```python
from build123d import *

# Parameters (mm, degrees)
SKETCH2_W           = 12
SKETCH2_H           = 40
BOSS_EXTRUDE1_DEPTH = 5
SKETCH3_W           = 12.004104261
SKETCH3_H           = 2.6
CUT_EXTRUDE1_DEPTH  = 15
SKETCH4_W           = 12
SKETCH4_H           = 4
BOSS_EXTRUDE2_DEPTH = 15
SKETCH5_R           = 3.75
CUT_EXTRUDE2_DEPTH  = 15


with BuildPart() as part:
    # Sketch2 → Boss-Extrude1 (new body)
    with BuildSketch(Plane(origin=(0, 0, 0), x_dir=(1, 0, 0), z_dir=(0, 1, 0))):
        with Locations((-9.764705882, 23.058823529)):
            Rectangle(SKETCH2_W, SKETCH2_H)
    extrude(amount=BOSS_EXTRUDE1_DEPTH)

    # Sketch3 → Cut-Extrude1 (cut)
    with BuildSketch(Plane.XY.offset(-3.058823529)):
        with Locations((-9.766758013, 2.489565118)):
            Rectangle(SKETCH3_W, SKETCH3_H)
    extrude(amount=-CUT_EXTRUDE1_DEPTH, mode=Mode.SUBTRACT)

    # Sketch4 → Boss-Extrude2 (add)
    with BuildSketch(Plane(origin=(0, 5, 0), x_dir=(1, 0, 0), z_dir=(0, 1, 0))):
        with Locations((-9.764705882, 41.058823529)):
            Rectangle(SKETCH4_W, SKETCH4_H)
    extrude(amount=BOSS_EXTRUDE2_DEPTH)

    # Sketch5 → Cut-Extrude2 (cut)
    with BuildSketch(Plane(origin=(0, 0, -43.058823529), x_dir=(-1, 0, 0), z_dir=(0, 0, -1))):
        with Locations((9.734798195, 13.917907096)):
            Circle(SKETCH5_R)
    extrude(amount=-CUT_EXTRUDE2_DEPTH, mode=Mode.SUBTRACT)


solid = part.part
```
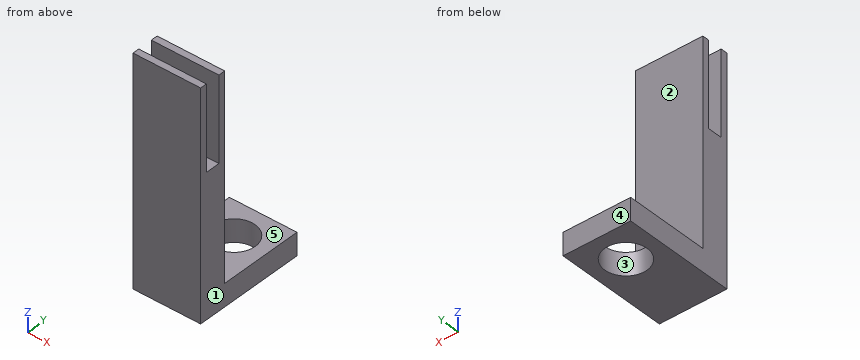
Verification items for the finished model (mm, model axes). Face numbers are marked on the shaded views. A direction names the side the tool comes from. Round coordinates to 2 decimals unless told otherwise and drop trailing zeros. Loops run counter-clockwise (first coordinate to the right, second up) from the corner with the lowest first, then second, coordinate; pieces in that order, holes last. Notation, with made-up numbers: (21.25, 56.25) -> (59.25, 56.25) arc R12 cw to (59.25, 77.25) -> close; hole circle Ø4 at (7, 35). An arc over 180 degrees is marked (long way). Answer as a JSON object with one key per item and string values.
Q1. Scan lines: line 1 (Y direction, x = -15, z = -12); line 2 (Y direction, x = -12.25, z = -30); line 3 (Z direction, x = -7.75, y = 9.25). Record each from-to range of solid material in increasing order. Write a range as from..to.
Data:
{"line 1": "y = 0..1.19, 3.79..5", "line 2": "y = 0..5", "line 3": "z = -43.06..-39.06"}
Q2. Section check B-B (x = -10.5). Record the boundary of the cut face in (y, z).
Data:
{"outline": "(0, -43.06) -> (10.25, -43.06) -> (10.25, -39.06) -> (5, -39.06) -> (5, -3.06) -> (3.79, -3.06) -> (3.79, -18.06) -> (1.19, -18.06) -> (1.19, -3.06) -> (0, -3.06) -> close; (17.59, -43.06) -> (20, -43.06) -> (20, -39.06) -> (17.59, -39.06) -> close"}
Q3. Section check A-A (z = -14). Record the boundary of the cut face in (x, y), then the cut area to 3 significant figures.
Data:
{"outline": "(-15.76, 0) -> (-3.76, 0) -> (-3.76, 1.19) -> (-15.76, 1.19) -> close; (-15.76, 3.79) -> (-3.76, 3.79) -> (-3.76, 5) -> (-15.76, 5) -> close", "area": "28.8 mm2"}
Q4. Go/stop test with flat-tipped pins: P1, Ø2, axis at x = -10, z = -29.5, coming from the +Y side; P2, Ø7, axis at x = -9.73, y = 13.92, coming from the -Z side; P3, Ø1.5, axis at x = -12.5, y = 11.5, coming from the +Z side; P4, Ø2, axis at x = -10.5, y = 2.5, coming from the +Z side. Record where each tip stops, or that it passes through.
Data:
{"P1": "stops at y = 5", "P2": "passes through", "P3": "stops at z = -39.06", "P4": "stops at z = -18.06"}
Q5. Draft check along Y on the marked faces 1, 2 and 3. Enter one of: pulls with the +Y half, pulls with the -Y half, needs draft (parallel to the pull), parting line crosses it, or undercut.
Data:
{"face 1": "needs draft", "face 2": "pulls with the +Y half", "face 3": "undercut"}
Q6. Section check D-D (x = -5.5). Record the boundary of the cut face in (y, z).
Data:
{"outline": "(0, -43.06) -> (20, -43.06) -> (20, -39.06) -> (5, -39.06) -> (5, -3.06) -> (3.79, -3.06) -> (3.79, -18.06) -> (1.19, -18.06) -> (1.19, -3.06) -> (0, -3.06) -> close"}
Q7. Section check C-C (y = 11.75). Record the boundary of the cut face in (x, z), then the cut area to 3 significant figures.
Data:
{"outline": "(-15.76, -43.06) -> (-12.79, -43.06) -> (-12.79, -39.06) -> (-15.76, -39.06) -> close; (-6.67, -43.06) -> (-3.76, -43.06) -> (-3.76, -39.06) -> (-6.67, -39.06) -> close", "area": "23.5 mm2"}
Q8. Access from +Z, -Z, +X, -X, +Y, -Y to the whole of each face (thin tool, end or side, straight path). Record for the marked faces 4 and 5.
Data:
{"face 4": "+Z, -Z, +X, -X, +Y", "face 5": "+Z, +X, -X, +Y"}
